```python
from build123d import *

# Parameters (mm, degrees)
SKETCH1_R           = 19
SKETCH1_R_2         = 4.75
BOSS_EXTRUDE1_DEPTH = 17
SKETCH2_R           = 1.25
CUT_EXTRUDE1_DEPTH  = 32.796226191
SKETCH3_R           = 1.6
CUT_EXTRUDE2_DEPTH  = 15
SKETCH4_R           = 11
SKETCH4_R_2         = 1.25
SKETCH4_R_3         = 4.75
CUT_EXTRUDE4_DEPTH  = 13
FILLET3_R           = 2


with BuildPart() as part:
    # Sketch1 → Boss-Extrude1 (new body)
    with BuildSketch(Plane(origin=(0, 0, 0), x_dir=(1, 0, 0), z_dir=(0, 1, 0))):
        with Locations(Location((0, 0, 0), (0, 0, 270))):
            Circle(SKETCH1_R)
        with Locations(Location((0, 0, 0), (0, 0, 270))):
            Circle(SKETCH1_R_2, mode=Mode.SUBTRACT)
    extrude(amount=BOSS_EXTRUDE1_DEPTH)

    # Sketch2 → Cut-Extrude1 (cut, through all)
    with BuildSketch(Plane(origin=(0, 17, 0), x_dir=(1, 0, 0), z_dir=(0, 1, 0))):
        with Locations(Location((-0.373838074, 7.25, 0), (0, 0, 270))):
            Circle(SKETCH2_R)
        with Locations(Location((7.25, 0.373838074, 0), (0, 0, 270))):
            Circle(SKETCH2_R)
        with Locations(Location((0.373838074, -7.25, 0), (0, 0, 270))):
            Circle(SKETCH2_R)
        with Locations(Location((-7.25, -0.373838074, 0), (0, 0, 270))):
            Circle(SKETCH2_R)
    extrude(amount=-CUT_EXTRUDE1_DEPTH, mode=Mode.SUBTRACT)

    # Sketch3 → Cut-Extrude2 (cut)
    with BuildSketch(Plane(origin=(0, 17, 0), x_dir=(1, 0, 0), z_dir=(0, 1, 0))):
        with Locations(Location((-0.373838074, 15, 0), (0, 0, 270))):
            Circle(SKETCH3_R)
        with Locations(Location((15, 0.373838074, 0), (0, 0, 270))):
            Circle(SKETCH3_R)
        with Locations(Location((0.373838074, -15, 0), (0, 0, 270))):
            Circle(SKETCH3_R)
        with Locations(Location((-15, -0.373838074, 0), (0, 0, 270))):
            Circle(SKETCH3_R)
    extrude(amount=-CUT_EXTRUDE2_DEPTH, mode=Mode.SUBTRACT)

    # Sketch4 → Cut-Extrude4 (cut)
    with BuildSketch(Plane(origin=(0, 17, 0), x_dir=(1, 0, 0), z_dir=(0, 1, 0))):
        with Locations(Location((0, 0, 0), (0, 0, 270))):
            Circle(SKETCH4_R)
        with Locations(Location((-0.373838074, 7.25, 0), (0, 0, 270))):
            Circle(SKETCH4_R_2, mode=Mode.SUBTRACT)
        with Locations(Location((0.373838074, -7.25, 0), (0, 0, 270))):
            Circle(SKETCH4_R_2, mode=Mode.SUBTRACT)
        with Locations(Location((0, 0, 0), (0, 0, 270))):
            Circle(SKETCH4_R_3, mode=Mode.SUBTRACT)
        with Locations(Location((-7.25, -0.373838074, 0), (0, 0, 270))):
            Circle(SKETCH4_R_2, mode=Mode.SUBTRACT)
        with Locations(Location((7.25, 0.373838074, 0), (0, 0, 270))):
            Circle(SKETCH4_R_2, mode=Mode.SUBTRACT)
    extrude(amount=-CUT_EXTRUDE4_DEPTH, mode=Mode.SUBTRACT)

    # Fillet3
    fillet3_edges = [part.edges().sort_by_distance(p)[0] for p in [
        (0, 17, -11),
        (0, 17, -19),
    ]]
    fillet(fillet3_edges, radius=FILLET3_R)


solid = part.part
```
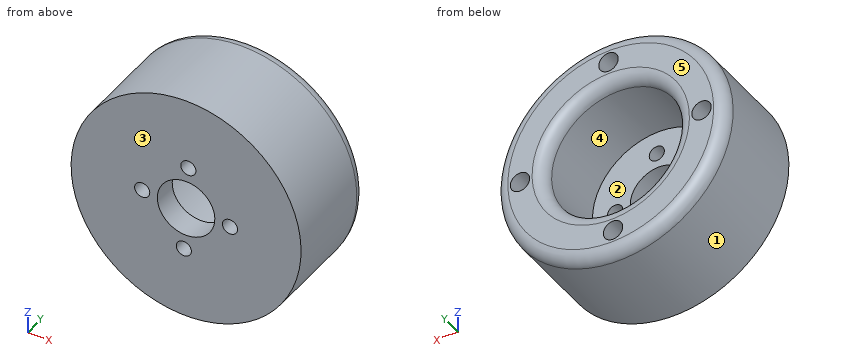
Input: part model. Units: mm. Frame: model coordinates. Face numbers are marked on the shaded views. A direction names the side the tool comes from. Give positions to 0.01 mm unless a question says otherwise; leave off trailing zeros. Loops run counter-clockwise (first coordinate to the right, second up) from the corner with the lowest first, then second, coordinate; pieces in that order, holes last. Notation, with made-up numbers: M 59,-20 L 106,-20 A20 cw 106,19 Z; hole C 64,61.25 d2. An arc over 180 degrees is marked long. Answer as CSV lines item,"result". Start each with the question number.
1. Section B-B on y = 7.5. Return loops of the section in (x, z).
2. Reachability of the marked faces 4 and 5 from +Z, -Z, +X, -X, +Y, -Y: full face, straight path, thin tool, end or side. Return the list, or none.
3. Pin query (flat end, axial travel): P1, Ø4, axis at y = 4.5, z = -1, coming from the -X side; P2, Ø5, axis at x = 14, z = -14.5, coming from the +Y side; P3, Ø1.6, axis at x = -15, z = 1, coming from the +Y side; P4, Ø2, axis at x = 7.25, z = -0.37, coming from the -Y side. Return the tip coordinate at first contact, or that it passes through.
4. Pull-direction query (Z, two-part tool) for the marked faces 1, 2 and 3; classes: released by +Z, released by -Z, zero draft, split by the parting line, or undercut.
5. Line query: L1, parallel to X at y = 6, z = 1; L2, parallel to X at y = 1.7, z = 0; L3, parallel to Z at x = -0.5, y = 12.5. Output: solid intervals per line, ascending.
6. Section A-A on z = 0. State how many separate pieces and enclosed holes the cut face has, plus the area to 3 significant figures.
Computed values:
1,outline,"C 0,0 d38; hole C -15,0.37 d3.2; hole C 0,0 d22; hole C -0.37,-15 d3.2; hole C 0.37,15 d3.2; hole C 15,-0.37 d3.2"
2,face 4,"+Y"
2,face 5,"+Z, -Z, +X, -X, +Y"
3,P1,"stops at x = -19"
3,P2,"stops at y = 16.89"
3,P3,"stops at y = 2"
3,P4,"passes through"
4,face 1,"split by the parting line"
4,face 2,"undercut"
4,face 3,"zero draft"
5,L1,"x = -18.97 to -16.47, -13.53 to -10.95, 10.95 to 14.18, 15.82 to 18.97"
5,L2,"x = -19 to -8.44, -6.06 to -4.75, 4.75 to 6.06, 8.44 to 19"
5,L3,"z = -18.99 to -16.6, -13.4 to -10.99, 10.99 to 13.66, 16.34 to 18.99"
6,separate pieces,"4"
6,enclosed holes,"0"
6,area,"206 mm²"
